Check sheet for the modelled part. Datum: model origin and axes. Units: mm. A direction names the side the tool comes from. Round coordinates to 2 decimals unless told otherwise and drop trailing zeros. Write each loop counter-clockwise with the first axis right and the second up, starting at its lowest first coordinate (ties: lowest second). Pieces come first, ordered by that corner, then holes. Notation, with made-up numbers: (49.5, 56) -> (90.5, 56) arc R19 cw to (90.5, 92) -> close; hole circle Ø8 at (-39.75, 51.25). An arc over 180 degrees is marked (long way). One line per item, written item: value. Start each with the question number.
Autodesk Inventor part; units mm, degrees
ref_plane "YZ Plane" through (0, 0, 0) normal (1, 0, 0) x (0, 1, 0)
ref_plane "XZ Plane" through (0, 0, 0) normal (0, 1, 0) x (-1, 0, 0)
ref_plane "XY Plane" through (0, 0, 0) normal (0, 0, 1) x (1, 0, 0)
sketch "スケッチ1" plane through (0, 0, 0) normal (0, 0, 1) x (1, 0, 0)
  line L0 (-14, 3.5) -> (-14, -3.5)
  line L1 (-14, -3.5) -> (-10.5, -3.5)
  line L2 (-10.5, -3.5) -> (-10.5, -3.4)
  line L3 (-10.5, -3.4) -> (-6.5, -3.4)
  line L4 (-6.5, -3.4) -> (-6.5, -3.5)
  line L5 (-6.5, -3.5) -> (-4, -3.5)
  line L6 (-4, -3.5) -> (-4, 3.5)
  line L7 (0, 0) -> (-14, 0) construction
  line L8 (0, 0) -> (0, 3.5) construction
  line L9 (-14, 3.5) -> (-10.5, 3.5)
  line L10 (-10.5, 3.5) -> (-10.5, 3.4)
  line L11 (-10.5, 3.4) -> (-6.5, 3.4)
  line L12 (-6.5, 3.4) -> (-6.5, 3.5)
  line L13 (-6.5, 3.5) -> (-4, 3.5)
  dimension "d0" = 0.1
  dimension "d1" = 7
  dimension "d2" = 4
  dimension "d3" = 14
  dimension "d4" = 3.5
  dimension "d5" = 2.5
revolve "回転1" add sketch "スケッチ1" angle 360 about axis through (0, 0, 0) along (0, 1, 0)
properties part number "Gbear_28_8" material "ステンレス鋼"
1. Cross-section at A-A (x = 0). Record the cut outline in (y, z), plus the area to 3 significant figures.
2. Cross-section at D-D (y = -2). Record the cut outline in (x, z), plus the area to 3 significant figures.
3. Material ranges on probe 1 along Z at (x, y) = (0, 3.45); probe 2 along X at (y, z) = (-0.25, -0.25); probe 3 along Z at (x, y) = (0, 1.5), recorded low to high.
4. Cross-section at C-C (x = 8.25). Record the cut outline in (y, z), plus the area to 3 significant figures.
5. Depth check by flat-ended pin: pin 1 Ø1 at (y, z) = (1.5, -4.5) entering from -X; pin 2 Ø4 at (y, z) = (-0.5, -11) entering from +X. Enter the tip coordinate at first touch or a pass-through.
6. Access from +Z, -Z, +X, -X, +Y, -Y to the whole of each face (thin tool, end or side, straight path). Record for faces 4 (the face through (0.867, 0.049, -3.905)), 5 (the face through (-5, -3.4, 5)).
7. Release check for a two-part mould opening along Z. For faces 1 (the face through (-5.1, 3.5, 9.4)), 2 (the face through (-12.932, -0.049, 5.362)), 3 (the face through (-5, 3.4, 5)) record: +Z half, -Z half, draft (parallel to the pull), parting line (faces both ways), or undercut.
8. Cross-section at B-B (z = 0). Record the cut outline in (x, y), plus the area to 3 significant figures.
Working result:
1. outline: (-3.5, -14) -> (3.5, -14) -> (3.5, -10.5) -> (3.4, -10.5) -> (3.4, -6.5) -> (3.5, -6.5) -> (3.5, -4) -> (-3.5, -4) -> (-3.5, -6.5) -> (-3.4, -6.5) -> (-3.4, -10.5) -> (-3.5, -10.5) -> close; (-3.5, 4) -> (3.5, 4) -> (3.5, 6.5) -> (3.4, 6.5) -> (3.4, 10.5) -> (3.5, 10.5) -> (3.5, 14) -> (-3.5, 14) -> (-3.5, 10.5) -> (-3.4, 10.5) -> (-3.4, 6.5) -> (-3.5, 6.5) -> close
1. area: 138 mm^2
2. outline: circle Ø28 at (0, 0); hole circle Ø8 at (0, 0)
2. area: 565 mm^2
3. probe 1: z = -14 to -10.5, -6.5 to -4, 4 to 6.5, 10.5 to 14
3. probe 2: x = -14 to -3.99, 3.99 to 14
3. probe 3: z = -14 to -4, 4 to 14
4. outline: (-3.5, -11.31) -> (3.5, -11.31) -> (3.5, -6.5) -> (3.4, -6.5) -> (3.4, 6.5) -> (3.5, 6.5) -> (3.5, 11.31) -> (-3.5, 11.31) -> (-3.5, 6.5) -> (-3.4, 6.5) -> (-3.4, -6.5) -> (-3.5, -6.5) -> close
4. area: 156 mm^2
5. pin 1: stops at x = -13.42
5. pin 2: stops at x = 10.72
6. face 4: +Y, -Y
6. face 5: -Y
7. face 1: draft
7. face 2: parting line
7. face 3: undercut
8. outline: (-14, -3.5) -> (-10.5, -3.5) -> (-10.5, -3.4) -> (-6.5, -3.4) -> (-6.5, -3.5) -> (-4, -3.5) -> (-4, 3.5) -> (-6.5, 3.5) -> (-6.5, 3.4) -> (-10.5, 3.4) -> (-10.5, 3.5) -> (-14, 3.5) -> close; (4, -3.5) -> (6.5, -3.5) -> (6.5, -3.4) -> (10.5, -3.4) -> (10.5, -3.5) -> (14, -3.5) -> (14, 3.5) -> (10.5, 3.5) -> (10.5, 3.4) -> (6.5, 3.4) -> (6.5, 3.5) -> (4, 3.5) -> close
8. area: 138 mm^2
